Verification items for the finished model (mm, model axes). Give positions to 0.01 mm unless a question says otherwise; leave off trailing zeros. Write each loop counter-clockwise with the first axis right and the second up, starting at its lowest first coordinate (ties: lowest second). Pieces come first, ordered by that corner, then holes.
Autodesk Inventor part; units mm, degrees
ref_plane "YZ Plane" through (0, 0, 0) normal (1, 0, 0) x (0, 1, 0)
ref_plane "XZ Plane" through (0, 0, 0) normal (0, 1, 0) x (-1, 0, 0)
ref_plane "XY Plane" through (0, 0, 0) normal (0, 0, 1) x (1, 0, 0)
sketch "Sketch1" plane through (0, 0, 0) normal (0, 0, 1) x (1, 0, 0)
  line L0 (-32.5001, -104.9789) -> (-32.5001, 105.0211)
  line L1 (-32.5001, -104.9789) -> (177.4999, -104.9789) construction
  line L2 (32.5001, -105) -> (32.5001, 105)
  line L3 (32.5001, -105) -> (242.5001, -105) construction
  arc A0 (32.5001, 105) -> (-32.5001, 105.0211) centre (0, 105.0211) ccw
  arc A1 (-32.5001, -104.9789) -> (32.5001, -105) centre (0, -104.9789) ccw
  line L4 (-37.5, -105) -> (-37.5, 105)
  line L5 (-37.5, -105) -> (172.5, -105) construction
  line L6 (37.5, -105) -> (37.5, 105)
  line L7 (37.5, -105) -> (247.5, -105) construction
  arc A2 (-37.5, -105) -> (37.5, -105) centre (0, -105) ccw
  arc A3 (37.5, 105) -> (-37.5, 105) centre (0, 105) ccw
  point P0 (0, 0)
  dimension "d0" = 210
  dimension "d1" = 90
  dimension "d2" = 210
  dimension "d3" = 90
  dimension "d4" = 210
  dimension "d5" = 90
  dimension "d6" = 210
  dimension "d7" = 90
extrude "Extrusion1" add sketch "Sketch1" along normal blind 10
sketch "Sketch3" plane through (0, 0, 10) normal (0, 0, 1) x (1, 0, 0)
  circle A0 centre (-35, 0) radius 1.5
  circle A1 centre (0, -140) radius 1.5
  circle A2 centre (35, 0) radius 1.5
  point P0 (0, 0)
  dimension "d11" = 3
  dimension "d12" = 3
  dimension "d13" = 3
hole "Hole1" at (-35, 0, 10) direction (0, 0, -1) diameter 3 end through all
sketch "Sketch5" plane through (0, 0, 10) normal (0, 0, 1) x (1, 0, 0)
  circle A0 centre (35, 0) radius 1.5
  point P0 (0, 0)
  dimension "d31" = 3
hole "Hole3" at (35, 0, 10) direction (0, 0, -1) diameter 3 end through all
sketch "Sketch6" plane through (0, 0, 10) normal (0, 0, 1) x (1, 0, 0)
  circle A0 centre (0, 140) radius 1.5
  point P0 (0, 0)
  dimension "d39" = 3
hole "Hole4" at (0, 140, 10) direction (0, 0, -1) diameter 3 end through all
properties part number "Chain"
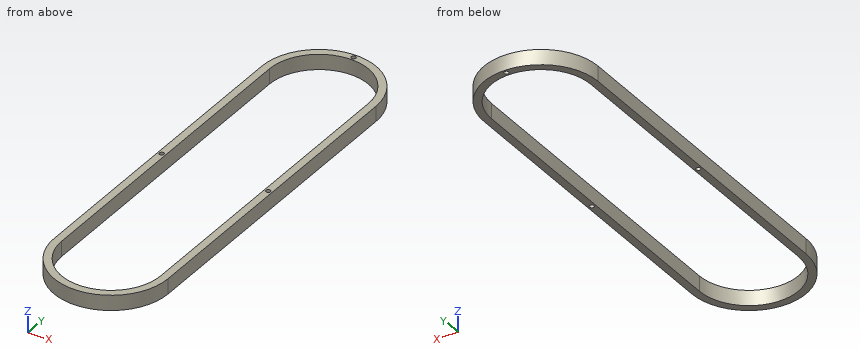
Item 1: Sectioned sample at A-A on z = 3.75. Record the cut outline in (x, y).
Answer key:
outline: (-37.5, -105) arc R37.5 ccw to (37.5, -105) - (37.5, 105) arc R37.5 ccw to (-37.5, 105) - close; hole circle Ø3 at (-35, 0); hole (-32.5, -104.98) arc R32.5 ccw to (32.5, -105) - (32.5, 105) arc R32.5 ccw to (-32.5, 105.02) - close; hole circle Ø3 at (0, 140); hole circle Ø3 at (35, 0)
Item 2: Depth check by flat-ended pin: pin 1 (6 mm diameter, centred on x = -26.5, z = 7, fed in from +Y); pin 2 (5 mm diameter, centred on x = -15, z = 7, fed in from -Y); pin 3 (3 mm diameter, centred on x = -0.5, z = 6.5, fed in from +Y). Enter the tip coordinate at first touch or a pass-through.
Answer key:
pin 1: stops at y = 134.22
pin 2: stops at y = -140.36
pin 3: stops at y = 142.5
Item 3: Sectioned sample at B-B on y = -29. Record the cut outline in (x, z).
Answer key:
outline: (-37.5, 0) - (-32.5, 0) - (-32.5, 10) - (-37.5, 10) - close; (32.5, 0) - (37.5, 0) - (37.5, 10) - (32.5, 10) - close
Item 4: Sectioned sample at C-C on x = -12.5. Record the cut outline in (y, z).
Answer key:
outline: (-140.36, 0) - (-134.98, 0) - (-134.98, 10) - (-140.36, 10) - close; (135.02, 0) - (140.36, 0) - (140.36, 10) - (135.02, 10) - close
Item 5: Scan lines: line 1 along X through (y, z) = (0, 7.25); line 2 along Y through (x, z) = (0, 2.5); line 3 along X through (y, z) = (-26.5, 7.5). Record each from-to range of solid material in increasing order.
Answer key:
line 1: x = -37.5 to -36.5, -33.5 to -32.5, 32.5 to 33.5, 36.5 to 37.5
line 2: y = -142.5 to -137.48, 137.52 to 138.5, 141.5 to 142.5
line 3: x = -37.5 to -32.5, 32.5 to 37.5
